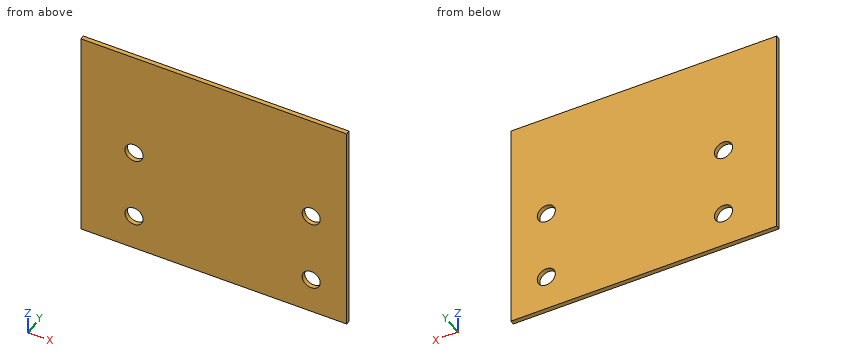
Autodesk Inventor part; units mm, degrees
ref_plane "YZ Plane" through (0, 0, 0) normal (1, 0, 0) x (0, 1, 0)
ref_plane "XZ Plane" through (0, 0, 0) normal (0, 1, 0) x (-1, 0, 0)
ref_plane "XY Plane" through (0, 0, 0) normal (0, 0, 1) x (1, 0, 0)
sketch "Sketch1" plane through (0, 0, 0) normal (0, 1, 0) x (-1, 0, 0)
  line L0 (0, 0) -> (95.25, 0)
  line L1 (95.25, 0) -> (95.25, 76.2)
  line L2 (95.25, 76.2) -> (0, 76.2)
  line L3 (0, 76.2) -> (0, 0)
  point P0 (76.2, 12.7)
  point P1 (12.7, 13.1017)
  point P2 (76.2, 38.1)
  point P3 (12.7, 38.1)
  dimension "d0" = 95.25
  dimension "d1" = 76.2
  dimension "d14" = 12.7
  dimension "d15" = 19.05
  dimension "d16" = 63.5
  dimension "d29" = 19.05
  dimension "d30" = 38.1
  dimension "d31" = 63.5
extrude "Extrusion2" add sketch "Sketch1" along normal blind 1.5875
sketch "Sketch3" plane through (0, 1.5875, 0) normal (0, 1, 0) x (1, 0, 0)
  line L0 (0, 0) -> (-95.25, 0)
  line L1 (-95.25, 0) -> (-95.25, -76.2)
  point P0 (-76.2, -12.7)
  point P1 (-12.7, -12.7)
  point P2 (-76.2, -38.1)
  point P3 (-12.7, -38.1)
  dimension "d19" = 19.05
  dimension "d20" = 12.7
  dimension "d21" = 63.5
  dimension "d32" = 25.4
  dimension "d33" = 63.5
  dimension "d34" = 19.05
hole "Hole3" at (-76.2, 1.5875, 12.7) at (-12.7, 1.5875, 12.7) at (-76.2, 1.5875, 38.1) at (-12.7, 1.5875, 38.1) direction (0, -1, 0) diameter 6.477 end through all
properties part number "slider"
Geometry check sheet. Reference: the model listing, model coordinates, mm. Give positions to 0.01 mm unless a question says otherwise; leave off trailing zeros. Write each loop counter-clockwise with the first axis right and the second up, starting at its lowest first coordinate (ties: lowest second). Pieces come first, ordered by that corner, then holes. Notation, with made-up numbers: (83.5, 77) - (127.5, 77) arc R12 ccw to (127.5, 84) - close; hole circle Ø7 at (-1.75, 61). An arc over 180 degrees is marked (long way). Use a Markdown table: item, result.
Q1. Go/stop test with a flat-tipped pin: P1, Ø5, axis at x = -12.7, z = 38.1, coming from the -Y side. Record where the tip stops, or that it passes through.
Computed:
| item | result |
|---|---|
| P1 | passes through |
Q2. Section check C-C, the plane y = 1.3. Enter the section's corners in (x, z).
Computed:
| item | result |
|---|---|
| outline | (-95.25, 0) - (0, 0) - (0, 76.2) - (-95.25, 76.2) - close; hole circle Ø6.48 at (-76.2, 12.7); hole circle Ø6.48 at (-76.2, 38.1); hole circle Ø6.48 at (-12.7, 12.7); hole circle Ø6.48 at (-12.7, 38.1) |
Q3. Section check A-A, the plane x = -76.2. Enter the section's corners in (y, z), then the cut area to 3 significant figures.
Computed:
| item | result |
|---|---|
| outline | (0, 0) - (1.59, 0) - (1.59, 9.46) - (0, 9.46) - close; (0, 15.94) - (1.59, 15.94) - (1.59, 34.86) - (0, 34.86) - close; (0, 41.34) - (1.59, 41.34) - (1.59, 76.2) - (0, 76.2) - close |
| area | 100 mm² |
Q4. Section check B-B, the plane z = 12.7. Enter the section's corners in (x, y), then the cut area to 3 significant figures.
Computed:
| item | result |
|---|---|
| outline | (-95.25, 0) - (-79.44, 0) - (-79.44, 1.59) - (-95.25, 1.59) - close; (-72.96, 0) - (-15.94, 0) - (-15.94, 1.59) - (-72.96, 1.59) - close; (-9.46, 0) - (0, 0) - (0, 1.59) - (-9.46, 1.59) - close |
| area | 131 mm² |
Q5. Thickness scan on L1, parallel to Z at x = -12.7, y = 0.9; L2, parallel to X at y = 0.55, z = 12.7. Record the ranges inside material, lowest first. Write a range as [from, to].
Computed:
| item | result |
|---|---|
| L1 | z = [0, 9.46], [15.94, 34.86], [41.34, 76.2] |
| L2 | x = [-95.25, -79.44], [-72.96, -15.94], [-9.46, 0] |
